```python
from build123d import *

# Parameters (mm, degrees)
F0_W     = 180
F0_H     = 40
F1_DEPTH = 5
F3_DEPTH = 25
F5_DEPTH = 25
F7_DEPTH = 25


with BuildPart() as f1:
    # F0 (on Top) → F1 (new body)
    with BuildSketch(Plane.XY):
        Rectangle(F0_W, F0_H)
    extrude(amount=F1_DEPTH)

    # F2 (on face) → F3 (cut)
    with BuildSketch(Plane.XY.offset(5)):
        Polygon((90, 20), (-90, 20), (90, 5), align=None)
    extrude(amount=-F3_DEPTH, mode=Mode.SUBTRACT)

    # F4 (on face) → F5 (cut)
    with BuildSketch(Plane.XY.offset(5)):
        Polygon((-75, 18.75), (-80, 19.1666666667), (-80, 0), (-75, 0), align=None)
        Polygon((80, 5.8333333333), (75, 6.25), (75, -7.5), (80, -7.5), align=None)
    extrude(amount=-F5_DEPTH, mode=Mode.SUBTRACT)

    # F6 (on face) → F7 (cut)
    with BuildSketch(Plane(origin=(0, 0, 0), x_dir=(1, 0, 0), z_dir=(0, 0, -1))):
        Polygon((-59.3428026841, -1.0552439201), (-69.2922490445, -2.0594934524), (-68.5892743718, -9.0241059046), (-58.6398280115, -8.0198563723), align=None)
        Polygon((70, 12), (60.0505536397, 10.9957504677), (60.7535283123, 4.0311380155), (70.7029746726, 5.0353875478), align=None)
    extrude(amount=-F7_DEPTH, mode=Mode.SUBTRACT)


solid = f1.part
```
The listing builds one solid part. Answer for the finished solid, in the listing's coordinates (mm). A direction names the side the tool comes from. Coordinates: 2 decimals unless noted, no trailing zeros. Loops run counter-clockwise (first coordinate to the right, second up) from the corner with the lowest first, then second, coordinate; pieces in that order, holes last. Notation, with made-up numbers: M -38,27 L 9,27 A29 ccw 9,62 Z; hole C -9.5,-36 d2. An arc over 180 degrees is marked long. Answer as CSV lines item,"result". Start each with the question number.
(1) The part is cut by section B-B (z = 4.25). Give the vertices of the cut face in (x, y), and give its area (3 significant figures).
(2) The part is cut by section C-C (x = -67). Give the vertices of the cut face in (y, z).
(3) The part is cut by section A-A (y = 15). Give the vertices of the cut face in (x, z), and give its area (3 significant figures).
(4) For faces 1 (the flat face through (77, -7.5, 3)), 2 (the flat face through (90, -8, 2)), 3 (the flat face through (65.659, -4.526, 2.465)), determine the directions among +Z, -Z, +X, -X, +Y, -Y from which every point of the face is accessible in a straight line to the end or side of a thin tool.
(5) The part is cut by section D-D (x = 34). Give the vertices of the cut face in (y, z).
(6) The mould has two halves that part along Y. Classify faces 4 (the flat face through (-90, 0, 2)), 5 (the flat face through (70.356, -8.469, 2.465)), 6 (the flat face through (84.93, 5.422, 2.535)), 7 (the flat face through (-1, -20, 2)): pulls with the +Y half, pulls with the -Y half, needs draft (parallel to the pull), parting line crosses it, or undercut.
(7) Given pin 1 (1.5 mm diameter, centred on x = -23, z = 3, fed in from +Y), flat-ended and moving along its own axis, determine where the tip first touches the part or whether it passes through.
(8) Find the intervals of material crossed by L1, parallel to X at y = 3.5, z = 2; L2, parallel to X at y = -1.5, z = 2.5; L3, parallel to Y at x = 78, z = 4.65, in increasing order. Write a range as [from, to].
Determined:
1,outline,"M -90,-20 L 90,-20 L 90,5 L 80,5.83 L 80,-7.5 L 75,-7.5 L 75,6.25 L -75,18.75 L -75,0 L -80,0 L -80,19.17 L -90,20 Z; hole M -69.29,2.06 L -59.34,1.06 L -58.64,8.02 L -68.59,9.02 Z; hole M 60.05,-11 L 70,-12 L 70.7,-5.04 L 60.75,-4.03 Z"
1,area,"5,550 mm2"
2,outline,"M -20,0 L 1.83,0 L 1.83,5 L -20,5 Z; M 8.86,0 L 18.08,0 L 18.08,5 L 8.86,5 Z"
3,outline,"M -90,0 L -80,0 L -80,5 L -90,5 Z; M -75,0 L -30,0 L -30,5 L -75,5 Z"
3,area,"275 mm2"
4,face 1,"+Z, -Z, +Y"
4,face 2,"+Z, -Z, +X, +Y, -Y"
4,face 3,"+Z, -Z"
5,outline,"M -20,0 L 9.67,0 L 9.67,5 L -20,5 Z"
6,face 4,"needs draft"
6,face 5,"undercut"
6,face 6,"pulls with the +Y half"
6,face 7,"pulls with the -Y half"
7,pin 1,"y = 14.48"
8,L1,"[-90, -80], [-75, -69.15], [-59.1, 75], [80, 90]"
8,L2,"[-90, 75], [80, 90]"
8,L3,"[-20, -7.5]"
